from build123d import *

# Parameters (mm, degrees)
SKETCH_1_R               = 200
EXTRUDE_1_DEPTH          = 100
EXTRUDE_1_DRAFT          = 30
SKETCH_4_R               = 325
EXTRUDE_2_DEPTH          = 10
FILLET_1_R               = 10
HOLE_WIZARD_M14_1_D      = 12
HOLE_WIZARD_1_D          = 21
PATTERN_CIRCULAR_1_COUNT = 12


# Read off the part's stored shape, not the designer's step: 抽壳1
with BuildPart() as part:
    # 草图1 → 凸台-拉伸1 (with draft: the straight prism first)
    with BuildSketch(Plane(origin=(0, 0, 0), x_dir=(1, 0, 0), z_dir=(0, 1, 0))):
        Circle(SKETCH_1_R)
    extrude(amount=-EXTRUDE_1_DEPTH)
    # 凸台-拉伸1: the draft: its side faces are tilted about the plane it starts from
    extrude_1_sides = [part.faces().sort_by_distance(p)[0] for p in [
        (-200, -50, 0),
    ]]
    draft(extrude_1_sides, Plane(origin=(0, 0, 0), x_dir=(1, 0, 0), z_dir=(0, 1, 0)), EXTRUDE_1_DRAFT)

    # 草图4 → 凸台-拉伸2 (add)
    with BuildSketch(Plane.XZ.offset(100)):
        with Locations(Location((0, 0, 0), (0, 0, 270))):
            Circle(SKETCH_4_R)
    extrude(amount=-EXTRUDE_2_DEPTH)

    # 抽壳1 outline → 抽壳1 (revolve, cut)
    with BuildSketch(Plane.XY):
        Polygon((246.188021535, -100), (194.226497308, -10), (0, -10), (0, -100), align=None)
    revolve(axis=Axis((0, 0, 0), (0, 1, 0)), mode=Mode.SUBTRACT)

    # 圆角1
    fillet_1_edges = [part.edges().sort_by_distance(p)[0] for p in [
        (-246.188021535, -100, 0),
        (-194.226497308, -10, 0),
        (-200, 0, 0),
        (-251.961524227, -90, 0),
    ]]
    fillet(fillet_1_edges, radius=FILLET_1_R)

    # M14 螺纹孔1 (through all)
    with Locations(Plane(origin=(0, -100, 0), x_dir=(-1, 0, 0), z_dir=(0, -1, 0))):
        with Locations((-110, -110), (-110, 110), (110, -110), (110, 110)):
            Hole(HOLE_WIZARD_M14_1_D / 2)

    # 孔1 (through all)
    with Locations(Plane(origin=(0, -90, 0), x_dir=(1, 0, 0), z_dir=(0, 1, 0))):
        with Locations((300, 0)):
            hole_wizard_1 = Hole(HOLE_WIZARD_1_D / 2)

    # 阵列(圆周)1: 孔1 ×12 about axis
    pattern_circular_1_axis = Axis((0, 0, 0), (0, 1, 0))
    for i in range(1, PATTERN_CIRCULAR_1_COUNT):
        add(hole_wizard_1.rotate(pattern_circular_1_axis, i * 360 / PATTERN_CIRCULAR_1_COUNT), mode=Mode.SUBTRACT)


solid = part.part
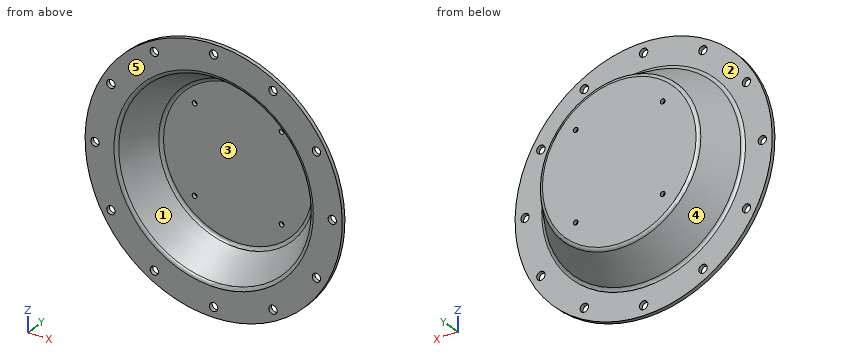
Design review of the part built by this model. Coordinates are the model's own, in mm. Face numbers are marked on the shaded views. A direction names the side the tool comes from. Round coordinates to 2 decimals unless told otherwise and drop trailing zeros. Write each loop counter-clockwise with the first axis right and the second up, starting at its lowest first coordinate (ties: lowest second). Pieces come first, ordered by that corner, then holes. Notation, with made-up numbers: M 57.25,8 L 102.25,8 A25 cw 102.25,24 Z; hole C 41.25,-14.5 d5. An arc over 180 degrees is marked long. One line per item, written item: value. Start each with the question number.
1. Take a section at C-C on y = -50. State the section outline as (x, z) points, then the cut area to 3 significant figures.
2. Take a section at A-A on x = -300. State the section outline as (y, z) points.
3. To check wall thickness, follow probe 1 along X at (y, z) = (-7, -110); probe 2 along Z at (x, y) = (110, -3). State the ranges of each line that lie inside material, in increasing order. Write a range as from..to.
4. For the marked faces 1 and 2, list the 3-axis set-ups (+Z, -Z, +X, -X, +Y, -Y) from which the entire face can be reached by the end or side of a thin tool; tool diameter is ignored.
5. Clearance check with flat-ended pins moving along their axes: P1, Ø8, axis at x = 40.5, y = -67, coming from the -Z side; P2, Ø2, axis at x = 165.5, y = -10.5, coming from the +Z side; P3, Ø1.5, axis at y = -73, z = 121.5, coming from the -X side. State where each tip first meets the part, or that it passes through.
6. Take a section at B-B on z = 300. State the section outline as (x, y) points, then the cut area to 3 significant figures.
7. Draft analysis for pull direction X (two halves, no side actions). For the marked faces 3, 4 and 5, state which applies: pulls with the +X half, pulls with the -X half, needs draft (parallel to the pull), parting line crosses it, or undercut.
Computed:
1. outline: C 0,0 d457.74; hole C 0,0 d434.64
1. area: 16,200 mm²
2. outline: M -100,-125 L -90,-125 L -90,-10.5 L -100,-10.5 Z; M -100,10.5 L -90,10.5 L -90,125 L -100,125 Z
3. probe 1: x = -171.85..-116, -104..104, 116..171.85
3. probe 2: z = -168.67..-116, -104..104, 116..168.67
4. face 1: -Y
4. face 2: +Y
5. P1: stops at z = -237.66
5. P2: stops at z = 124.41
5. P3: stops at x = -210.12
6. outline: M -125,-100 L -10.5,-100 L -10.5,-90 L -125,-90 Z; M 10.5,-100 L 125,-100 L 125,-90 L 10.5,-90 Z
6. area: 2,290 mm²
7. face 3: undercut
7. face 4: parting line crosses it
7. face 5: needs draft
